Autodesk Inventor part; units mm, degrees
ref_plane "YZ Plane" through (0, 0, 0) normal (1, 0, 0) x (0, 1, 0)
ref_plane "XZ Plane" through (0, 0, 0) normal (0, 1, 0) x (-1, 0, 0)
ref_plane "XY Plane" through (0, 0, 0) normal (0, 0, 1) x (1, 0, 0)
sketch "Sketch1" plane through (0, 0, 0) normal (0, 0, 1) x (1, 0, 0)
  line L0 (-55.5, 90) -> (55.5, 90)
  line L1 (67.5, 78) -> (67.5, -78)
  line L2 (55.5, -90) -> (-55.5, -90)
  line L3 (-67.5, -78) -> (-67.5, 78)
  line L4 (-37.5, 50) -> (37.5, 50)
  line L5 (37.5, 50) -> (37.5, -50)
  line L6 (37.5, -50) -> (-37.5, -50)
  line L7 (-37.5, -50) -> (-37.5, 50)
  arc A0 (-55.5, 90) -> (-67.5, 78) centre (-55.5, 78) ccw
  arc A1 (67.5, 78) -> (55.5, 90) centre (55.5, 78) ccw
  arc A2 (55.5, -90) -> (67.5, -78) centre (55.5, -78) ccw
  arc A3 (-67.5, -78) -> (-55.5, -90) centre (-55.5, -78) ccw
  point P0 (0, 0)
  point P1 (-67.5, 90)
  point P2 (67.5, -90)
  point P3 (67.5, 90)
  point P4 (-67.5, -90)
  dimension "d0" = 180
  dimension "d2" = 100
  dimension "d3" = 40
  dimension "d4" = 40
  dimension "d7" = 30
  dimension "d8" = 30
  dimension "d10" = 75
  dimension "d11" = 12
  dimension "d21" = 37.5
  dimension "d22" = 50
extrude "Extrusion1" add sketch "Sketch1" along normal blind 5
sketch "Sketch3" plane through (0, 0, 5) normal (0, 0, 1) x (1, 0, 0)
  line L0 (55.5, 90) -> (-55.5, 90) construction
  line L1 (0, 90) -> (0, -90) construction
  line L2 (-55.5, -90) -> (55.5, -90) construction
  line L3 (-67.5, 78) -> (-67.5, -78) construction
  line L4 (-67.5, 0) -> (67.5, 0) construction
  line L5 (67.5, -78) -> (67.5, 78) construction
  point P0 (0, 0)
  point P1 (-52.5, 75)
  point P2 (52.5, 75)
  point P3 (52.5, -75)
  point P4 (-52.5, -75)
  dimension "d12" = 15
  dimension "d13" = 15
hole "Hole1" at (-52.5, 75, 5) at (52.5, 75, 5) at (52.5, -75, 5) at (-52.5, -75, 5) direction (0, 0, -1) diameter 7 end through all
sketch "Sketch4" plane through (0, 0, 5) normal (0, 0, 1) x (1, 0, 0)
  line L0 (-55.5, -90) -> (55.5, -90)
  line L1 (67.5, -78) -> (67.5, 78)
  point P0 (0, 0)
  point P1 (0, -70)
  dimension "d23" = 20
  dimension "d24" = 67.5
hole "Hole2" at (0, -70, 5) direction (0, 0, -1) diameter 2 depth 1
equation "\"d3\" = d4"
equation "\"d8\" = d7"
properties part number "TapaBC" material "MDF Medium Density Fiberboard"
Build history of the part. All positions in model axes, mm. A direction names the side the tool comes from. Coordinates: 2 decimals unless noted, no trailing zeros. Write each loop counter-clockwise with the first axis right and the second up, starting at its lowest first coordinate (ties: lowest second). Pieces come first, ordered by that corner, then holes.
1. Band-saw the part on B-B, the plane y = -75. Give the cut face in (x, z), and give its area (3 significant figures).
Answer block:
outline: (-67.5, 0) - (-56, 0) - (-56, 5) - (-67.5, 5) - close; (-49, 0) - (49, 0) - (49, 5) - (-49, 5) - close; (56, 0) - (67.5, 0) - (67.5, 5) - (56, 5) - close
area: 605 mm2
2. 3-axis set-ups, long thin cutter, end or side, ignore diameter. For faces 1 (the flat face through (-37.5, -1, 2)), 2 (the flat face through (44, 1, 5)): which of +Z, -Z, +X, -X, +Y, -Y reach the whole face in a straight line?
Answer block:
face 1: +Z, -Z
face 2: +Z, +X, -X, +Y, -Y
3. Pull direction Y, two halves, no side cores. Call faces 3 (the cylindrical face through (49.55, -76.88, 2.46)), 4 (the flat face through (1, -90, 2)), 5 (the flat face through (-67.5, -1, 2)): released by +Y, released by -Y, zero draft, split by the parting line, or undercut.
Answer block:
face 3: undercut
face 4: released by -Y
face 5: zero draft
4. Band-saw the part on A-A, the plane x = -34. Give the cut face in (y, z), and give its area (3 significant figures).
Answer block:
outline: (-90, 0) - (-50, 0) - (-50, 5) - (-90, 5) - close; (50, 0) - (90, 0) - (90, 5) - (50, 5) - close
area: 400 mm2
5. Band-saw the part on C-C, the plane z = 2.65. Give the cut face in (x, y).
Answer block:
outline: (-67.5, -78) arc R12 ccw to (-55.5, -90) - (55.5, -90) arc R12 ccw to (67.5, -78) - (67.5, 78) arc R12 ccw to (55.5, 90) - (-55.5, 90) arc R12 ccw to (-67.5, 78) - close; hole circle Ø7 at (-52.5, -75); hole circle Ø7 at (-52.5, 75); hole (-37.5, -50) - (37.5, -50) - (37.5, 50) - (-37.5, 50) - close; hole circle Ø7 at (52.5, -75); hole circle Ø7 at (52.5, 75)
6. Drill centre lines: probe 1 along Y at (x, z) = (52.5, 3.85); probe 2 along X at (y, z) = (-75, 3.2); probe 3 along X at (y, z) = (-40, 4.3). Where is each one in solid material? Low to high.
Answer block:
probe 1: y = -90 to -78.5, -71.5 to 71.5, 78.5 to 90
probe 2: x = -67.5 to -56, -49 to 49, 56 to 67.5
probe 3: x = -67.5 to -37.5, 37.5 to 67.5
7. Drop a flat-ended pin along its axis: pin 1 (5.5 mm diameter, centred on x = -52.5, y = 75, fed in from +Z). Give the stop position or say it passes through.
Answer block:
pin 1: passes through
8. Band-saw the part on D-D, the plane x = -52.5. Give the cut face in (y, z).
Answer block:
outline: (-90, 0) - (-78.5, 0) - (-78.5, 5) - (-90, 5) - close; (-71.5, 0) - (71.5, 0) - (71.5, 5) - (-71.5, 5) - close; (78.5, 0) - (90, 0) - (90, 5) - (78.5, 5) - close
